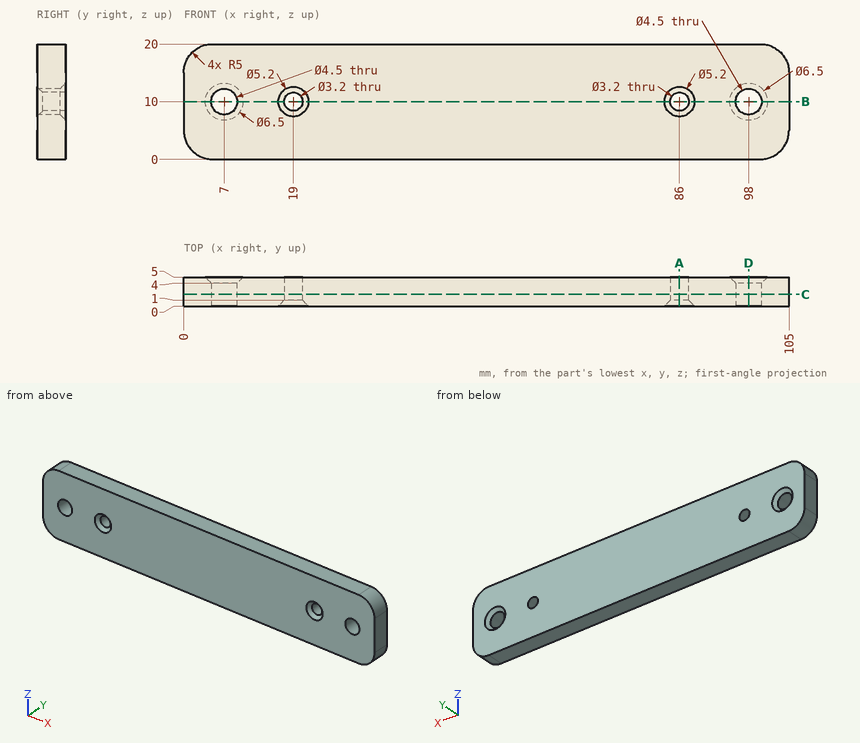
Part print with two shaded views. Sizes in mm from the minimum x, y, z corner. Give positions to 0.01 mm unless a question says otherwise; leave off trailing zeros. Order: outer loops, then holes, each group sorted by start corner. A loop starts at its lowest first (then second) coordinate and runs counter-clockwise, first axis right, second up.
(1) Drill centre lines: L1, parallel to X at y = 3.6, z = 10; L2, parallel to Z at x = 86, y = 3.9; L3, parallel to Z at x = 98, y = 1.4. Where is each one in solid material? Low to high.
(2) Saw through at D-D, the plane x = 98. Give the cut face in (y, z).
(3) Saw through at A-A, the plane x = 86. Give the cut face in (y, z), then the cut area to 3 significant figures.
(4) Flat gauge pins, fed straight in: pin 1 (3.5 mm diameter, centred on x = 19, z = 10, fed in from -Y); pin 2 (5 mm diameter, centred on x = 98, z = 10, fed in from +Y). Where does each tip first touch, or does it go through?
(5) Saw through at C-C, the plane y = 2.05. Give the cut face in (x, z).
(6) Saw through at B-B, the plane z = 10. Give the cut face in (x, y).
Results found:
1. L1: x = 0 to 4.75, 9.25 to 17.4, 20.6 to 84.4, 87.6 to 95.75, 100.25 to 105
1. L2: z = 0 to 8.4, 11.6 to 20
1. L3: z = 0 to 7.75, 12.25 to 20
2. outline: (0, 0) - (5, 0) - (5, 6.75) - (4, 7.75) - (0, 7.75) - close; (0, 12.25) - (4, 12.25) - (5, 13.25) - (5, 20) - (0, 20) - close
3. outline: (0, 0) - (5, 0) - (5, 8.4) - (1, 8.4) - (0, 7.4) - close; (0, 12.6) - (1, 11.6) - (5, 11.6) - (5, 20) - (0, 20) - close
3. area: 83.0 mm2
4. pin 1: stops at y = 0.85
4. pin 2: stops at y = 4.25
5. outline: (0, 5) arc R5 ccw to (5, 0) - (100, 0) arc R5 ccw to (105, 5) - (105, 15) arc R5 ccw to (100, 20) - (5, 20) arc R5 ccw to (0, 15) - close; hole circle Ø4.5 at (7, 10); hole circle Ø3.2 at (19, 10); hole circle Ø3.2 at (86, 10); hole circle Ø4.5 at (98, 10)
6. outline: (0, 0) - (4.75, 0) - (4.75, 4) - (3.75, 5) - (0, 5) - close; (9.25, 0) - (16.4, 0) - (17.4, 1) - (17.4, 5) - (10.25, 5) - (9.25, 4) - close; (20.6, 1) - (21.6, 0) - (83.4, 0) - (84.4, 1) - (84.4, 5) - (20.6, 5) - close; (87.6, 1) - (88.6, 0) - (95.75, 0) - (95.75, 4) - (94.75, 5) - (87.6, 5) - close; (100.25, 0) - (105, 0) - (105, 5) - (101.25, 5) - (100.25, 4) - close
